Geometry: final body of the model. Coordinates: model frame, mm. Face numbers are marked on the shaded views. A direction names the side the tool comes from. Round coordinates to 2 decimals unless told otherwise and drop trailing zeros. Loops run counter-clockwise (first coordinate to the right, second up) from the corner with the lowest first, then second, coordinate; pieces in that order, holes last. Notation, with made-up numbers: M -39,-1 L 2,-1 A23 cw 2,35 Z; hole C -39.5,-21 d4. An arc over 180 degrees is marked long. Answer as a JSON object with one key per item and string values.
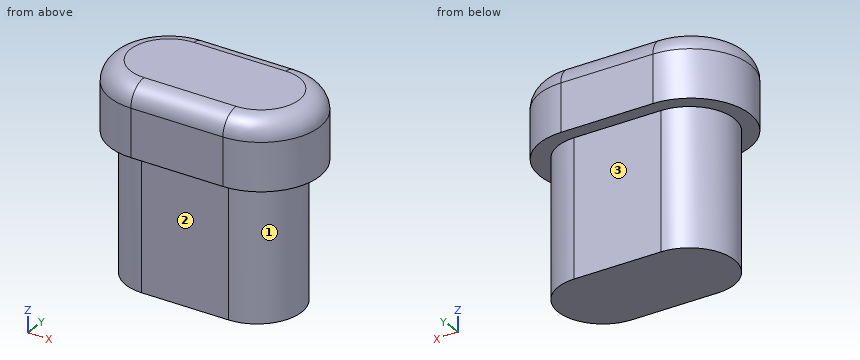
```python
from build123d import *

# Parameters (mm, degrees)
PAD_DEPTH    = 20
PAD001_DEPTH = 10
FILLET_R     = 3


with BuildPart() as part:
    # Sketch → Pad (new body)
    with BuildSketch(Plane.XY):
        with BuildLine():
            ThreePointArc((-6.5, 6.5), (-13, 0), (-6.5, -6.5))
            Line((-6.5, -6.5), (6.5, -6.5))
            ThreePointArc((6.5, -6.5), (13, 0), (6.5, 6.5))
            Line((-6.5, 6.5), (6.5, 6.5))
        make_face()
    extrude(amount=PAD_DEPTH)

    # Sketch001 (on Face6 of Pad) → Pad001 (join)
    with BuildSketch(Plane.XY.offset(20)):
        with BuildLine():
            ThreePointArc((-6.716935, 8.602443), (-15.319378, 0), (-6.716935, -8.602443))
            Line((-6.716935, -8.602443), (7.081573, -8.602443))
            ThreePointArc((7.081573, -8.602443), (15.684016, 0), (7.081573, 8.602443))
            Line((-6.716935, 8.602443), (7.081573, 8.602443))
        make_face()
    extrude(amount=PAD001_DEPTH)

    # Fillet
    fillet_edges = [part.edges().sort_by_distance(p)[0] for p in [
        (0.182319, 8.602443, 30),
        (-15.319378, 0, 30),
        (0.182319, -8.602443, 30),
        (15.684016, 0, 30),
    ]]
    fillet(fillet_edges, radius=FILLET_R)


solid = part.part
```
1) Set-up query: the marked faces 1, 2 and 3. Return all of +Z, -Z, +X, -X, +Y, -Y with unobstructed straight access to the full face (end or side cutting, diameter ignored); none if empty.
Geometry results:
{"face 1": "-Z, +X", "face 2": "-Z, +X, -X, -Y", "face 3": "-Z, +X, -X, +Y"}
2) Cut plane B-B on x = -4. Return the cut outline in (y, z), and give its area (3 significant figures).
Geometry results:
{"outline": "M -8.6,20 L -6.5,20 L -6.5,0 L 6.5,0 L 6.5,20 L 8.6,20 L 8.6,27 A3 ccw 5.6,30 L -5.6,30 A3 ccw -8.6,27 Z", "area": "428 mm2"}
3) Cut plane D-D on z = 7.25. Return the cut outline in (x, y), and give its area (3 significant figures).
Geometry results:
{"outline": "M -6.5,-6.5 L 6.5,-6.5 A6.5 ccw 6.5,6.5 L -6.5,6.5 A6.5 ccw Z", "area": "302 mm2"}
4) Cut plane A-A on y = 0. Return the cut outline in (x, z), and give its area (3 significant figures).
Geometry results:
{"outline": "M -15.32,20 L -13,20 L -13,0 L 13,0 L 13,20 L 15.68,20 L 15.68,27 A3 ccw 12.68,30 L -12.32,30 A3 ccw -15.32,27 Z", "area": "826 mm2"}
5) Cut plane C-C on z = 25.5. Return the cut outline in (x, y).
Geometry results:
{"outline": "M -6.72,-8.6 L 7.08,-8.6 A8.6 ccw 7.08,8.6 L -6.72,8.6 A8.6 ccw Z"}
6) First-contact query: pin 1 (4 mm diameter, centred on x = 1.5, z = 10, fed in from +Y); pin 2 (1 mm diameter, centred on x = -5, z = 8.5, fed in from -Y); pin 3 (1.5 mm diameter, centred on y = -2.5, z = 17.5, fed in from -X). Flat tips, straight axial feed; report the tip coordinate or a pass-through.
Geometry results:
{"pin 1": "y = 6.5", "pin 2": "y = -6.5", "pin 3": "x = -12.76"}
7) Line query: probe 1 along Y at (x, z) = (1, 14); probe 2 along Z at (x, y) = (-11.5, -4.5); probe 3 along Y at (x, z) = (13.5, 22.25). Output: solid intervals per line, ascending.
Geometry results:
{"probe 1": "-6.5 to 6.5", "probe 2": "20 to 29.84", "probe 3": "-5.73 to 5.73"}
